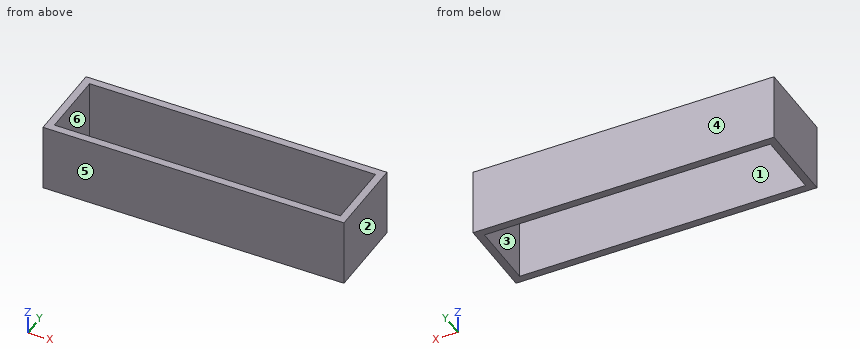
from build123d import *

# Parameters (mm, degrees)
SKETCH1_W               = 200
SKETCH1_H               = 45
BOSS_EXTRUDE1_DEPTH     = 55
CUT_EXTRUDE1_DEPTH      = 213.249852768
CUT_EXTRUDE1_DEPTH_BACK = 213.249852768
SKETCH2_W               = 190
SKETCH2_H               = 45


with BuildPart() as part:
    # Sketch1 → Boss-Extrude1 (new body)
    with BuildSketch(Plane(origin=(0, 0, 0), x_dir=(1, 0, 0), z_dir=(0, 1, 0))):
        with Locations((100, 22.5)):
            Rectangle(SKETCH1_W, SKETCH1_H)
    extrude(amount=BOSS_EXTRUDE1_DEPTH)

    # Sketch2 → Cut-Extrude1 (cut, two sides: drawn at the far end of the back side and taken through both)
    with BuildSketch(Plane.XY.offset(-CUT_EXTRUDE1_DEPTH_BACK)):
        with Locations((100, 27.5)):
            Rectangle(SKETCH2_W, SKETCH2_H)
    extrude(amount=CUT_EXTRUDE1_DEPTH + CUT_EXTRUDE1_DEPTH_BACK, mode=Mode.SUBTRACT)


solid = part.part
Geometry check sheet. Reference: the model listing, model coordinates, mm. Face numbers are marked on the shaded views. A direction names the side the tool comes from. Round coordinates to 2 decimals unless told otherwise and drop trailing zeros. Order: outer loops, then holes, each group sorted by start corner. A loop starts at its lowest first (then second) coordinate and runs counter-clockwise, first axis right, second up. Notation, with made-up numbers: M -21.5,-15.5 L 14.5,-15.5 A12 ccw 14.5,-9.5 Z; hole C 1,89 d2. An arc over 180 degrees is marked long. Write each question's results on one line, items separated by ' | '. Start each with the question number.
1. Cross-section at C-C on z = -7. Record the boundary of the cut face in (x, y).
2. Material ranges on L1, parallel to X at y = 25.5, z = -42; L2, parallel to Y at x = 119, z = -31, recorded low to high. Write a range as from..to.
3. Cross-section at B-B on y = 47. Record the boundary of the cut face in (x, z), plus the area to 3 significant figures.
4. Go/stop test with a flat-tipped pin: P1, Ø10, axis at x = 57.5, z = -23.5, coming from the -Y side. Record where the tip stops, or that it passes through.
5. Draft check along X on the marked faces 1, 2, 3 and 4. Enter one of: pulls with the +X half, pulls with the -X half, needs draft (parallel to the pull), parting line crosses it, or undercut.
6. Set-up check for the marked faces 5 and 6: record each of +Z, -Z, +X, -X, +Y, -Y from which the full face is reachable in a straight line by a thin tool's end or side.
7. Cross-section at A-A on x = 120.5. Record the boundary of the cut face in (y, z).
Resolved:
1) outline: M 0,0 L 200,0 L 200,55 L 0,55 Z; hole M 5,5 L 195,5 L 195,50 L 5,50 Z
2) L1: 0..5, 195..200 | L2: 0..5, 50..55
3) outline: M 0,-45 L 5,-45 L 5,0 L 0,0 Z; M 195,-45 L 200,-45 L 200,0 L 195,0 Z | area: 450 mm2
4) P1: y = 0
5) face 1: undercut | face 2: pulls with the +X half | face 3: undercut | face 4: needs draft
6) face 5: +Z, -Z, +X, -X, -Y | face 6: +Z, -Z
7) outline: M 0,-45 L 5,-45 L 5,0 L 0,0 Z; M 50,-45 L 55,-45 L 55,0 L 50,0 Z
